Solid Edge part; units mm, degrees
sketch "Sketch1" plane through (0, 0, 0) normal (0, -1, 0) x (1, 0, 0)
  arc A0 (-6.7188, -2.4454) -> (-8.9271, -3.2492) centre (-7.5737, -3.5322) ccw
  arc A1 (0, 9.5) -> (0, 7.15) centre (0.7155, 8.325) ccw
  arc A2 (0, 9.5) -> (-8.9271, -3.2492) centre (0, 0) cw
  arc A3 (0, 7.15) -> (-6.7188, -2.4454) centre (0, 0) cw
extrude "Protrusion1" add sketch "Sketch1" against normal blind 1
sketch "Sketch2" plane through (0, 0, 0) normal (0, -1, 0) x (1, 0, 0)
  line L0 (12.2182, -5.5033) -> (8.9416, -3.209)
  line L1 (8.9416, -3.209) -> (6.0737, -7.3048)
  line L2 (6.0737, -7.3048) -> (9.3503, -9.5991)
  line L3 (9.3503, -9.5991) -> (12.2182, -5.5033)
extrude "Henkel_1" add sketch "Sketch2" against normal blind 1
sketch "Sketch3" plane through (0, 0, 0) normal (0, -1, 0) x (1, 0, 0)
  line L0 (10.5799, -4.3562) -> (7.712, -8.4519)
  line L1 (9.3503, -9.5991) -> (7.712, -8.4519)
  line L2 (12.2182, -5.5033) -> (9.3503, -9.5991)
  line L3 (10.5799, -4.3562) -> (12.2182, -5.5033)
extrude "Henkel_2" add sketch "Sketch3" against normal blind 3
fillet "Verrundung_1" radius 1 3 edges at (8.9416, 0.5, -3.209) (6.0737, 0.5, -7.3048) (9.146, 1, -6.4041)
Work out the finished part from the listing and answer in its coordinate system (mm). A direction names the side the tool comes from. Give positions to 0.01 mm unless a question says otherwise; leave off trailing zeros. Loops run counter-clockwise (first coordinate to the right, second up) from the corner with the lowest first, then second, coordinate; pieces in that order, holes last. Notation, with made-up numbers: M -36,65 L -26,65 A17 ccw -26,80 Z; hole C 48.25,-20 d6. An arc over 180 degrees is marked long. One line per item, written item: value. Start each with the question number.
1. Determine the mould class of faces 1 (the face through (-0.66, 0.49, 8.34)), 2 (the face through (-8.028, 0.493, -2.226)), 3 (the face through (10, 3, -7)), 4 (the face through (5.729, 0.493, -4.278)) for opening direction Z: released by +Z, released by -Z, zero draft, split by the parting line, or undercut.
2. Each of these flat-tipped pins is pushed along its axis until it touches: P1, Ø1.5, axis at y = 2.5, z = -1, coming from the -X side; P2, Ø9.5, axis at x = -0.5, z = -4, coming from the +Y side. Where does it stop, or does it pass through?
3. Which of the six approach directions +Z, -Z, +X, -X, +Y, -Y give full straight-line access (tool end or side, diameter ignored) to faces 5 (the face through (9.166, 2.493, -6.375)), 6 (the face through (10.764, 1.479, -7.58)), 7 (the face through (7.994, 0.493, -8.649))?
4. Find section B-B (z = 0). Give the vertices of the cut face in (x, y).
5. Find section D-D (z = 4.5). Give the vertices of the cut face in (x, y).
6. Find section A-A (x = 5.75). Give the vertices of the cut face in (y, z).
7. Find the intervals of material crossed by probe 1 along Z at (x, y) = (0, 0.7); probe 2 along Y at (x, z) = (3.75, -7.5); probe 3 along X at (y, z) = (0.6, 0), in increasing order.
Reported:
1. face 1: undercut
1. face 2: released by +Z
1. face 3: zero draft
1. face 4: undercut
2. P1: passes through
2. P2: stops at y = 1
3. face 5: +Z, -X, +Y
3. face 6: -Z, +X, +Y, -Y
3. face 7: -Z, +Y, -Y
4. outline: M 7.15,0 L 9.5,0 L 9.5,1 L 7.15,1 Z
5. outline: M 5.56,0 L 8.37,0 L 8.37,1 L 5.56,1 Z
6. outline: M 0,-7.61 L 1,-7.61 L 1,-4.25 L 0,-4.25 Z; M 0,4.25 L 1,4.25 L 1,7.56 L 0,7.56 Z
7. probe 1: z = -9.5 to -7.15, 7.15 to 9.5
7. probe 2: y = 0 to 1
7. probe 3: x = 7.15 to 9.5
